```python
from build123d import *

# Parameters (mm, degrees)
F1_DEPTH = 25.4


with BuildPart() as f1:
    # F0 (on Top) → F1 (new body)
    with BuildSketch(Plane.XY):
        with BuildLine():
            Line((-19.949808, -14.713609), (-20.223535, -14.713609))
            Line((-20.223535, -14.713609), (-20.223535, -28.192073))
            Line((-20.223535, -28.192073), (-18.638604, -28.192073))
            Line((-18.638604, -28.192073), (-15.463604, -28.192073))
            Line((-15.463604, -28.192073), (-13.878673, -28.192073))
            Line((-13.878673, -28.192073), (-13.878673, -14.713609))
            Line((-13.878673, -14.713609), (-14.1524, -14.713609))
            ThreePointArc((-14.1524, -14.713609), (-16.063492, -15.580491), (-16.670104, -17.589415))
            Line((-16.670104, -17.589415), (-15.463604, -26.635145))
            Line((-15.463604, -26.635145), (-18.638604, -26.635145))
            Line((-18.638604, -26.635145), (-17.432104, -17.589415))
            ThreePointArc((-17.432104, -17.589415), (-18.038716, -15.580491), (-19.949808, -14.713609))
        make_face()
        with BuildLine():
            Line((-18.638604, -28.192073), (-20.223535, -28.192073))
            Line((-20.223535, -28.192073), (-20.223535, -40.113609))
            Line((-20.223535, -40.113609), (-19.949808, -40.113609))
            ThreePointArc((-19.949808, -40.113609), (-18.038716, -39.246728), (-17.432104, -37.237803))
            Line((-17.432104, -37.237803), (-18.638604, -28.192073))
        make_face()
        with BuildLine():
            Line((-13.878673, -28.192073), (-15.463604, -28.192073))
            Line((-15.463604, -28.192073), (-16.670104, -37.237803))
            ThreePointArc((-16.670104, -37.237803), (-16.063492, -39.246728), (-14.1524, -40.113609))
            Line((-14.1524, -40.113609), (-13.878673, -40.113609))
            Line((-13.878673, -40.113609), (-13.878673, -28.192073))
        make_face()
    extrude(amount=F1_DEPTH)


solid = f1.part
```
Work out the finished part from the listing and answer in its coordinate system (mm). A direction names the side the tool comes from. Give positions to 0.01 mm unless a question says otherwise; leave off trailing zeros. Order: outer loops, then holes, each group sorted by start corner. A loop starts at its lowest first (then second) coordinate and runs counter-clockwise, first axis right, second up. Notation, with made-up numbers: M 54.5,63 L 95.5,63 A31 cw 95.5,91 Z; hole C -12,82 d11. An arc over 180 degrees is marked long. Return JSON: item names as keys, results as strings.
1) Section D-D, the plane y = -28.75 is taken. Write down the section's boundary in (x, z), plus the area to 3 significant figures.
Resolved:
{"outline": "M -20.22,0 L -18.56,0 L -18.56,25.4 L -20.22,25.4 Z; M -15.54,0 L -13.88,0 L -13.88,25.4 L -15.54,25.4 Z", "area": "84.3 mm^2"}
2) Straight lines are drawn through the part: line 1 along X through (y, z) = (-29.25, 6.5); line 2 along X through (y, z) = (-31.5, 7.25); line 3 along Y through (x, z) = (-19.25, 13.75). For each, find the intervals that lie inside material, in ascending order. Write a range as [from, to].
Resolved:
{"line 1": "[-20.22, -18.5], [-15.6, -13.88]", "line 2": "[-20.22, -18.2], [-15.9, -13.88]", "line 3": "[-40.02, -14.81]"}
3) Each of these flat-tipped pins is pushed along its axis until it touches: pin 1 (1.6 mm diameter, centred on x = -17.5, z = 16, fed in from +Y); pin 2 (3 mm diameter, centred on x = -14.5, z = 18.5, fed in from +Y). Where does it stop, or does it pass through?
Resolved:
{"pin 1": "y = -15.32", "pin 2": "y = -14.71"}
4) Section B-B, the plane z = 19.5 is taken. Write down the section's boundary in (x, y).
Resolved:
{"outline": "M -20.22,-40.11 L -19.95,-40.11 A2.54 ccw -17.43,-37.24 L -18.64,-28.19 L -15.46,-28.19 L -16.67,-37.24 A2.54 ccw -14.15,-40.11 L -13.88,-40.11 L -13.88,-14.71 L -14.15,-14.71 A2.54 ccw -16.67,-17.59 L -15.46,-26.64 L -18.64,-26.64 L -17.43,-17.59 A2.54 ccw -19.95,-14.71 L -20.22,-14.71 Z"}
5) For a pull along X with two mould halves and no side action, classify faces 1 (the flat face through (-20.224, -27, 13)), 2 (the flat face through (-13.879, -28, 13)), 3 (the cylindrical face through (-16.043, -15.558, 12.522)) as +X half, -X half, draft (parallel to the pull), parting line (faces both ways), or undercut.
Resolved:
{"face 1": "-X half", "face 2": "+X half", "face 3": "undercut"}
6) Section A-A, the plane y = -38 is taken. Write down the section's boundary in (x, z).
Resolved:
{"outline": "M -20.22,0 L -17.45,0 L -17.45,25.4 L -20.22,25.4 Z; M -16.66,0 L -13.88,0 L -13.88,25.4 L -16.66,25.4 Z"}
7) A tool of negligible diameter and unlimited length cuts with its end or side. For faces 4 (the flat face through (-18.027, -32.778, 12.522)), 5 (the flat face through (-17, -27, 0)), from which of +Z, -Z, +X, -X, +Y, -Y can it reach the whole face along a straight path? Write none if from no direction.
Resolved:
{"face 4": "+Z, -Z", "face 5": "-Z, +X, -X, +Y, -Y"}
8) Section C-C, the plane x = -17.75 is taken. Write down the section's boundary in (y, z).
Resolved:
{"outline": "M -38.84,0 L -34.85,0 L -34.85,25.4 L -38.84,25.4 Z; M -28.19,0 L -26.64,0 L -26.64,25.4 L -28.19,25.4 Z; M -19.97,0 L -15.98,0 L -15.98,25.4 L -19.97,25.4 Z"}
